```python
from build123d import *

# Parameters (mm, degrees)
SKETCH1_R           = 1.5
SKETCH1_R_2         = 7.75
BOSS_EXTRUDE1_DEPTH = 3
FILLET1_R           = 3
SKETCH2_R           = 1
CUT_EXTRUDE1_DEPTH  = 10


with BuildPart() as part:
    # Sketch1 → Boss-Extrude1 (new body)
    with BuildSketch(Plane.XY):
        Polygon((7.989824602, 62), (-7.989824602, 62), (-20.5, 47.899715907), (-20.5, 17.599715907), (-11, 0), (0, 0), (11, 0), (20.5, 17.599715907), (20.5, 47.899715907), align=None)
        with Locations((-6, 4)):
            Circle(SKETCH1_R, mode=Mode.SUBTRACT)
        with Locations((-13.5, 37.599715907)):
            Circle(SKETCH1_R, mode=Mode.SUBTRACT)
        with Locations((-5.239824602, 58)):
            Circle(SKETCH1_R, mode=Mode.SUBTRACT)
        with Locations(Location((5.239824602, 58, 0), (0, 0, 180))):
            Circle(SKETCH1_R, mode=Mode.SUBTRACT)
        with Locations(Location((13.5, 37.599715907, 0), (0, 0, 180))):
            Circle(SKETCH1_R, mode=Mode.SUBTRACT)
        with Locations(Location((6, 4, 0), (0, 0, 180))):
            Circle(SKETCH1_R, mode=Mode.SUBTRACT)
        with Locations((7.5, 17.599715907)):
            Circle(SKETCH1_R_2, mode=Mode.SUBTRACT)
        with BuildLine():
            Line((8.730303993, 36.099715907), (-8.730303993, 36.099715907))
            ThreePointArc((-8.730303993, 36.099715907), (-10.179901517, 33.861140502), (-12.574074074, 32.686197699))
            Line((-12.574074074, 32.686197699), (-12.574074074, 17.599715907))
            Line((-12.574074074, 17.599715907), (-12.52949298, 17.599715907))
            Line((-12.52949298, 17.599715907), (-12.52949298, 23.253614409))
            Line((-12.52949298, 23.253614409), (-3.75, 23.253614409))
            Line((-3.75, 23.253614409), (-3.75, 17.599715907))
            ThreePointArc((-3.75, 17.599715907), (1.043381087, 26.812455576), (11.338812838, 28.174497985))
            ThreePointArc((11.338812838, 28.174497985), (14.402792388, 29.760560356), (12.574074074, 32.686197699))
            ThreePointArc((12.574074074, 32.686197699), (10.179901517, 33.861140502), (8.730303993, 36.099715907))
        make_face(mode=Mode.SUBTRACT)
        with BuildLine():
            Line((8.730303993, 39.099715907), (-8.730303993, 39.099715907))
            ThreePointArc((-8.730303993, 39.099715907), (-10.179901517, 41.338291312), (-12.574074074, 42.513234115))
            ThreePointArc((-12.574074074, 42.513234115), (0, 51.099715907), (12.574074074, 42.513234115))
            ThreePointArc((12.574074074, 42.513234115), (10.179901517, 41.338291312), (8.730303993, 39.099715907))
        make_face(mode=Mode.SUBTRACT)
    extrude(amount=BOSS_EXTRUDE1_DEPTH)

    # Fillet1
    fillet1_edges = [part.edges().sort_by_distance(p)[0] for p in [
        (-11, 0, 1.5),
        (-20.5, 17.599715907, 1.5),
        (-20.5, 47.899715907, 1.5),
        (-7.989824602, 62, 1.5),
        (7.989824602, 62, 1.5),
        (20.5, 47.899715907, 1.5),
        (20.5, 17.599715907, 1.5),
        (11, 0, 1.5),
    ]]
    fillet(fillet1_edges, radius=FILLET1_R)

    # Sketch2 → Cut-Extrude1 (cut)
    with BuildSketch(Plane.XY.offset(3)):
        with Locations((16.960133769, 18.410352932)):
            Circle(SKETCH2_R)
        with Locations((-10.808600311, 17.213150766)):
            Circle(SKETCH2_R)
    extrude(amount=-CUT_EXTRUDE1_DEPTH, mode=Mode.SUBTRACT)


solid = part.part
```
CAD build for the part. Positions are in the model's coordinates, mm. A direction names the side the tool comes from. Round coordinates to 2 decimals unless told otherwise and drop trailing zeros. Write each loop counter-clockwise with the first axis right and the second up, starting at its lowest first coordinate (ties: lowest second). Pieces come first, ordered by that corner, then holes. Notation, with made-up numbers: (33, 1.5) - (76, 1.5) arc R31 cw to (76, 35.5) - close; hole circle Ø11 at (48, -38.75). An arc over 180 degrees is marked (long way). Write item = value, one per line. Start each with the question number.
Q1. Probe L1, parallel to Y at x = -9, z = 1.9; L2, parallel to Y at x = 13.5, z = 1.3; L3, parallel to Y at x = 1.5, z = 2.8. List the from-to ranges inside material, lowest first. Write a range as from..to.
Q2. Drop flat-ended pins along their axis: pin 1 (3 mm diameter, centred on x = 16.96, y = 18.41, fed in from +Z); pin 2 (1.5 mm diameter, centred on x = -14.5, z = 1, fed in from +Y); pin 3 (1 mm diameter, centred on y = 6.5, z = 2, fed in from -X). Give the stop position or say it passes through.
Q3. Which spindle directions (+Z, -Z, +X, -X, +Y, -Y) get a long thin tool onto all of the face, cutting with end or side? Do faces 4 (the cylindrical face through (10.208, 33.836, 1.479)), 5 (the flat face through (-20.5, 33, 1)). Say none if no direction does.
Q4. Band-saw the part on C-C (x = 6). Give the cut face in (y, z).
Q5. Band-saw the part on B-B (y = 4). Give the cut face in (x, z).
Q6. Band-saw the part on D-D (y = 46). Give the cut face in (x, z), then the cut area to 3 significant figures.
Q7. Mould opens along Y. For faces 1 (the cylindrical face through (-20.41, 17.63, 1.52)), 2 (the cylindrical face through (-20.3, 47.84, 1.52)), 3 (the flat face through (0, 39.1, 1)) say: pulls with the +Y half, pulls with the -Y half, needs draft (parallel to the pull), parting line crosses it, or undercut.
Q8. Band-saw the part on A-A (x = -3). Give the cut face in (y, z), then the cut area to 3 significant figures.
Answers below:
q1.L1 = 0..23.25, 35.42..39.78, 47.66..60.86
q1.L2 = 4.63..12.69, 22.51..28.47, 32.29..36.1, 39.1..55.79
q1.L3 = 0..12.69, 22.51..27.12, 36.1..39.1, 51.02..62
q2.pin_1 = 3
q2.pin_2 = 55.51
q2.pin_3 = -14.78
q3.face_4 = +Z, -Z
q3.face_5 = +Z, -Z, -X, +Y, -Y
q4.outline = (0, 0) - (2.5, 0) - (2.5, 3) - (0, 3) - close; (5.5, 0) - (10, 0) - (10, 3) - (5.5, 3) - close; (25.2, 0) - (28.75, 0) - (28.75, 3) - (25.2, 3) - close; (36.1, 0) - (39.1, 0) - (39.1, 3) - (36.1, 3) - close; (49.69, 0) - (56.71, 0) - (56.71, 3) - (49.69, 3) - close; (59.29, 0) - (62, 0) - (62, 3) - (59.29, 3) - close
q5.outline = (-13.16, 0) - (-7.5, 0) - (-7.5, 3) - (-13.16, 3) - close; (-4.5, 0) - (4.5, 0) - (4.5, 3) - (-4.5, 3) - close; (7.5, 0) - (13.16, 0) - (13.16, 3) - (7.5, 3) - close
q6.outline = (-20.5, 0) - (-10.57, 0) - (-10.57, 3) - (-20.5, 3) - close; (10.57, 0) - (20.5, 0) - (20.5, 3) - (10.57, 3) - close
q6.area = 59.6 mm2
q7.face_1 = pulls with the -Y half
q7.face_2 = pulls with the +Y half
q7.face_3 = undercut
q8.outline = (0, 0) - (21.64, 0) - (21.64, 3) - (0, 3) - close; (36.1, 0) - (39.1, 0) - (39.1, 3) - (36.1, 3) - close; (50.76, 0) - (62, 0) - (62, 3) - (50.76, 3) - close
q8.area = 108 mm2
